Verification items for the finished model (mm, model axes). Face numbers are marked on the shaded views. A direction names the side the tool comes from. Round coordinates to 2 decimals unless told otherwise and drop trailing zeros. Order: outer loops, then holes, each group sorted by start corner. A loop starts at its lowest first (then second) coordinate and runs counter-clockwise, first axis right, second up. Notation, with made-up numbers: (88.5, 29.5) -> (143.5, 29.5) arc R10 ccw to (143.5, 39.5) -> close; hole circle Ø7 at (69.5, -13.75). An arc over 180 degrees is marked (long way). Put each result on its own line as item: value.
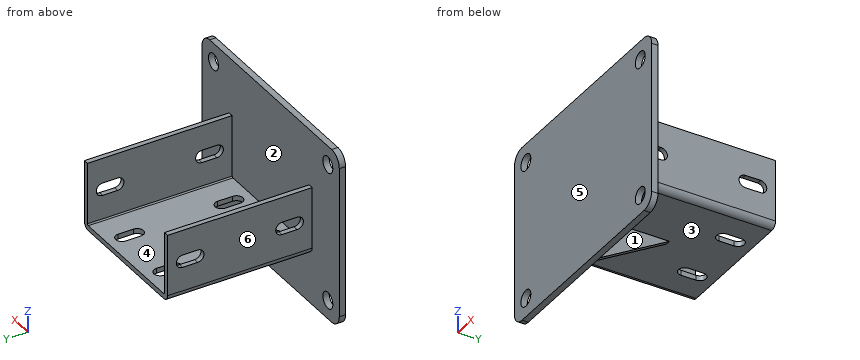
```python
from build123d import *

# Parameters (mm, degrees)
SKETCH_2_W          = 180
SKETCH_2_H          = 140
EXTRUDE_1_DEPTH     = 5
EXTRUDE_1_2_DEPTH   = 115
EXTRUDE_2_DEPTH     = 2
CUT_EXTRUDE_1_DEPTH = 145.5
SKETCH_6_R          = 6.5
CUT_EXTRUDE_2_DEPTH = 6
FILLET_1_R          = 10
CUT_EXTRUDE_3_REACH = 101


with BuildPart() as part:
    # Эскиз2 → Extrude 1 (new body)
    with BuildSketch(Plane(origin=(0, 0, 0), x_dir=(1, 0, 0), z_dir=(0, 1, 0))):
        Rectangle(SKETCH_2_W, SKETCH_2_H)
    extrude(amount=EXTRUDE_1_DEPTH)

    # Эскиз3 → Extrude 1 2 (add)
    with BuildSketch(Plane(origin=(0, 5, 0), x_dir=(1, 0, 0), z_dir=(0, 1, 0))):
        with BuildLine():
            Line((-50.5, -25), (-50.5, 24))
            ThreePointArc((-50.5, 24), (-50.207106781, 24.707106781), (-49.5, 25))
            Line((-49.5, 25), (49.5, 25))
            ThreePointArc((49.5, 25), (50.207106781, 24.707106781), (50.5, 24))
            Line((50.5, 24), (50.5, -25))
            Line((50.5, -25), (54.5, -25))
            Line((54.5, -25), (54.5, 24))
            ThreePointArc((54.5, 24), (53.035533906, 27.535533906), (49.5, 29))
            Line((49.5, 29), (-49.5, 29))
            ThreePointArc((-49.5, 29), (-53.035533906, 27.535533906), (-54.5, 24))
            Line((-54.5, 24), (-54.5, -25))
            Line((-54.5, -25), (-50.5, -25))
        make_face()
    extrude(amount=EXTRUDE_1_2_DEPTH)

    # Эскиз4 → Бобышка-Вытянуть2 (add, symmetric)
    with BuildSketch(Plane(origin=(0, 0, 0), x_dir=(0, 0, -1), z_dir=(1, 0, 0))):
        Polygon((29, 67.353829072), (65, 5), (29, 5), align=None)
    extrude(amount=EXTRUDE_2_DEPTH, both=True)

    # Эскиз5 → Вырез-Вытянуть1 (cut, through all)
    with BuildSketch(Plane(origin=(54.5, 0, 0), x_dir=(0, 0, -1), z_dir=(1, 0, 0))):
        with BuildLine():
            Line((5, 108), (5, 96))
            ThreePointArc((5, 96), (0, 91), (-5, 96))
            Line((-5, 96), (-5, 108))
            ThreePointArc((-5, 108), (0, 113), (5, 108))
        make_face()
        with BuildLine():
            Line((5, 29), (5, 17))
            ThreePointArc((5, 17), (0, 12), (-5, 17))
            Line((-5, 17), (-5, 29))
            ThreePointArc((-5, 29), (0, 34), (5, 29))
        make_face()
    extrude(amount=-CUT_EXTRUDE_1_DEPTH, mode=Mode.SUBTRACT)

    # Эскиз6 → Вырез-Вытянуть2 (cut, through all)
    with BuildSketch(Plane(origin=(0, 5, 0), x_dir=(1, 0, 0), z_dir=(0, 1, 0))):
        with Locations(Location((-75, 55, 0), (0, 0, 270))):  # turned: the seam where the file's is
            Circle(SKETCH_6_R)
        with Locations(Location((-75, -55, 0), (0, 0, 270))):  # turned: the seam where the file's is
            Circle(SKETCH_6_R)
        with Locations(Location((75, 55, 0), (0, 0, 270))):  # turned: the seam where the file's is
            Circle(SKETCH_6_R)
        with Locations(Location((75, -55, 0), (0, 0, 270))):  # turned: the seam where the file's is
            Circle(SKETCH_6_R)
    extrude(amount=-CUT_EXTRUDE_2_DEPTH, mode=Mode.SUBTRACT)

    # Скругление1
    fillet_1_edges = [part.edges().sort_by_distance(p)[0] for p in [
        (90, 2.5, 70),
        (-90, 2.5, 70),
        (-90, 2.5, -70),
        (90, 2.5, -70),
    ]]
    fillet(fillet_1_edges, radius=FILLET_1_R)

    # Эскиз8 → Вырез-Вытянуть3 (cut, up to next)
    with BuildSketch(Plane(origin=(0, 0, -29), x_dir=(-1, 0, 0), z_dir=(0, 0, -1)), mode=Mode.PRIVATE) as cut_extrude_3_sk1:
        with BuildLine():
            Line((-20, 108), (-20, 96))
            ThreePointArc((-20, 96), (-25, 91), (-30, 96))
            Line((-30, 96), (-30, 108))
            ThreePointArc((-30, 108), (-25, 113), (-20, 108))
        make_face()
    cut_extrude_3_tool1 = extrude(cut_extrude_3_sk1.sketch, amount=-CUT_EXTRUDE_3_REACH, mode=Mode.PRIVATE) & part.part
    add(cut_extrude_3_tool1.solids().sort_by_distance((25, 102, -29))[0], mode=Mode.SUBTRACT)
    # Эскиз8 → Вырез-Вытянуть3 (cut, up to next)
    with BuildSketch(Plane(origin=(0, 0, -29), x_dir=(-1, 0, 0), z_dir=(0, 0, -1)), mode=Mode.PRIVATE) as cut_extrude_3_sk2:
        with BuildLine():
            Line((-20, 29), (-20, 17))
            ThreePointArc((-20, 17), (-25, 12), (-30, 17))
            Line((-30, 17), (-30, 29))
            ThreePointArc((-30, 29), (-25, 34), (-20, 29))
        make_face()
    cut_extrude_3_tool2 = extrude(cut_extrude_3_sk2.sketch, amount=-CUT_EXTRUDE_3_REACH, mode=Mode.PRIVATE) & part.part
    add(cut_extrude_3_tool2.solids().sort_by_distance((25, 23, -29))[0], mode=Mode.SUBTRACT)
    # Эскиз8 → Вырез-Вытянуть3 (cut, up to next)
    with BuildSketch(Plane(origin=(0, 0, -29), x_dir=(-1, 0, 0), z_dir=(0, 0, -1)), mode=Mode.PRIVATE) as cut_extrude_3_sk3:
        with BuildLine():
            Line((20, 108), (20, 96))
            ThreePointArc((20, 96), (25, 91), (30, 96))
            Line((30, 96), (30, 108))
            ThreePointArc((30, 108), (25, 113), (20, 108))
        make_face()
    cut_extrude_3_tool3 = extrude(cut_extrude_3_sk3.sketch, amount=-CUT_EXTRUDE_3_REACH, mode=Mode.PRIVATE) & part.part
    add(cut_extrude_3_tool3.solids().sort_by_distance((-25, 102, -29))[0], mode=Mode.SUBTRACT)
    # Эскиз8 → Вырез-Вытянуть3 (cut, up to next)
    with BuildSketch(Plane(origin=(0, 0, -29), x_dir=(-1, 0, 0), z_dir=(0, 0, -1)), mode=Mode.PRIVATE) as cut_extrude_3_sk4:
        with BuildLine():
            Line((20, 29), (20, 17))
            ThreePointArc((20, 17), (25, 12), (30, 17))
            Line((30, 17), (30, 29))
            ThreePointArc((30, 29), (25, 34), (20, 29))
        make_face()
    cut_extrude_3_tool4 = extrude(cut_extrude_3_sk4.sketch, amount=-CUT_EXTRUDE_3_REACH, mode=Mode.PRIVATE) & part.part
    add(cut_extrude_3_tool4.solids().sort_by_distance((-25, 23, -29))[0], mode=Mode.SUBTRACT)


solid = part.part
```
Item 1: Depth check by flat-ended pin: pin 1 Ø2 at (y, z) = (23, -26.5) entering from +X; pin 2 Ø1.2 at (y, z) = (101.5, -26.5) entering from -X; pin 3 Ø3 at (x, y) = (-52.5, 102) entering from +Z; pin 4 Ø17 at (x, z) = (75, -55) entering from -Y. Enter the tip coordinate at first touch or a pass-through.
Geometry check:
pin 1: x = 54.27
pin 2: x = -54.12
pin 3: z = 25
pin 4: y = 0
Item 2: Material ranges on line 1 along X through (y, z) = (3.1, -55); line 2 along Z through (x, y) = (29.5, 43.5); line 3 along Y through (x, z) = (66.5, -52), recorded low to high.
Geometry check:
line 1: -90 to -81.5, -68.5 to 68.5, 81.5 to 90
line 2: -29 to -25
line 3: 0 to 5
Item 3: Sectioned sample at A-A, the plane z = 0. Record the boundary of the cut face in (x, y), then the cut area to 3 significant figures.
Geometry check:
outline: (-90, 0) -> (90, 0) -> (90, 5) -> (54.5, 5) -> (54.5, 12) -> (50.5, 12) -> (50.5, 5) -> (-50.5, 5) -> (-50.5, 12) -> (-54.5, 12) -> (-54.5, 5) -> (-90, 5) -> close; (-54.5, 34) -> (-50.5, 34) -> (-50.5, 91) -> (-54.5, 91) -> close; (-54.5, 113) -> (-50.5, 113) -> (-50.5, 120) -> (-54.5, 120) -> close; (50.5, 34) -> (54.5, 34) -> (54.5, 91) -> (50.5, 91) -> close; (50.5, 113) -> (54.5, 113) -> (54.5, 120) -> (50.5, 120) -> close
area: 1,470 mm2
Item 4: Tool access check on the marked faces 1, 2 and 3. Record the directions out of +Z, -Z, +X, -X, +Y, -Y that give a thin tool (end or side, any length) a straight path to the whole face; none if there is none.
Geometry check:
face 1: -Z, +X, +Y
face 2: +Y
face 3: -Z, +Y
Item 5: Sectioned sample at D-D, the plane z = 55. Record the boundary of the cut face in (x, y), then the cut area to 3 significant figures.
Geometry check:
outline: (-90, 0) -> (-81.5, 0) -> (-81.5, 5) -> (-90, 5) -> close; (-68.5, 0) -> (68.5, 0) -> (68.5, 5) -> (-68.5, 5) -> close; (81.5, 0) -> (90, 0) -> (90, 5) -> (81.5, 5) -> close
area: 770 mm2
Item 6: Sectioned sample at C-C, the plane y = 101.5. Record the boundary of the cut face in (x, z).
Geometry check:
outline: (-54.5, -24) arc R5 ccw to (-49.5, -29) -> (-30, -29) -> (-30, -25) -> (-49.5, -25) arc R1 cw to (-50.5, -24) -> (-50.5, -5) -> (-54.5, -5) -> close; (-54.5, 5) -> (-50.5, 5) -> (-50.5, 25) -> (-54.5, 25) -> close; (-20, -29) -> (20, -29) -> (20, -25) -> (-20, -25) -> close; (30, -29) -> (49.5, -29) arc R5 ccw to (54.5, -24) -> (54.5, -5) -> (50.5, -5) -> (50.5, -24) arc R1 cw to (49.5, -25) -> (30, -25) -> close; (50.5, 5) -> (54.5, 5) -> (54.5, 25) -> (50.5, 25) -> close
Item 7: Sectioned sample at B-B, the plane x = 75. Record the boundary of the cut face in (y, z), then the cut area to 3 significant figures.
Geometry check:
outline: (0, -70) -> (5, -70) -> (5, -61.5) -> (0, -61.5) -> close; (0, -48.5) -> (5, -48.5) -> (5, 48.5) -> (0, 48.5) -> close; (0, 61.5) -> (5, 61.5) -> (5, 70) -> (0, 70) -> close
area: 570 mm2
Item 8: Release check for a two-part mould opening along X. For the marked faces 4, 5 and 6 record: pulls with the +X half, pulls with the -X half, needs draft (parallel to the pull), parting line crosses it, or undercut.
Geometry check:
face 4: undercut
face 5: needs draft
face 6: pulls with the -X half
